Could you check a few things on this model? Use its own coordinates, in mm. A direction names the side the tool comes from. Round coordinates to 2 decimals unless told otherwise and drop trailing zeros. Loops run counter-clockwise (first coordinate to the right, second up) from the corner with the lowest first, then second, coordinate; pieces in that order, holes last.
from build123d import *

# Parameters (mm, degrees)
F1_DEPTH       = 19
F3_D           = 3.4
F3_CSINK_D     = 6.72
F3_CSINK_ANGLE = 90
F5_DEPTH       = 25
F6_R           = 2


with BuildPart() as f1:
    # F0 (on Front) → F1 (new body)
    with BuildSketch(Plane.XZ):
        Polygon((0, 5.0361528993), (0, 0), (40, 0), (40, 10), (35, 10), (35, 5.0361528993), align=None)
    extrude(amount=F1_DEPTH)

    # F3 (through all)
    with Locations(Plane(origin=(0, 0, 0), x_dir=(1, 0, 0), z_dir=(0, 0, -1))):
        with Locations((9, 12), (29, 12)):
            CounterSinkHole(F3_D / 2, F3_CSINK_D / 2, counter_sink_angle=F3_CSINK_ANGLE)

    # F4 (on face) → F5 (cut)
    with BuildSketch(Plane(origin=(0, 0, 0), x_dir=(1, 0, 0), z_dir=(0, 0, -1))):
        Polygon((40, 3.5), (5, 0), (40, 0), align=None)
    extrude(amount=-F5_DEPTH, mode=Mode.SUBTRACT)

    # F6
    f6_edges = [f1.edges().sort_by_distance(p)[0] for p in [
        (40, -11.25, 0),
    ]]
    fillet(f6_edges, radius=F6_R)


solid = f1.part
Item 1: If we section it at D-D, the plane x = 9: Please give me the cut outline in (y, z).
Results list:
outline: (-19, 0) - (-15.36, 0) - (-13.7, 1.66) - (-13.7, 5.04) - (-19, 5.04) - close; (-10.3, 1.66) - (-8.64, 0) - (-0.4, 0) - (-0.4, 5.04) - (-10.3, 5.04) - close
Item 2: Will these pins go through, and if not, where does the flat tip stop? pin 1 (3 mm diameter, centred on y = -9.5, z = 7, fed in from -X); pin 2 (4.5 mm diameter, centred on x = 29, y = -12, fed in from -Z); pin 3 (5.5 mm diameter, centred on x = 19.5, y = -7, fed in from +Z).
Results list:
pin 1: stops at x = 35
pin 2: stops at z = 1.11
pin 3: stops at z = 5.04
Item 3: We'd pull the mould along X, two halves only. Please class faces 3 (the cylindrical face through (27.43, -11.35, 3.37)), 4 (the flat face through (0, -9, 3)), 5 (the flat face through (38, -11, 10)), 6 (the flat face through (40, -11, 6)): released by +X, released by -X, zero draft, split by the parting line, or undercut.
Results list:
face 3: undercut
face 4: released by -X
face 5: zero draft
face 6: released by +X
Item 4: If we section it at B-B, the plane z = 2.5: Please give me the cut outline in (x, y), then the cut area to 3 significant figures.
Results list:
outline: (0, -19) - (40, -19) - (40, -3.5) - (5, 0) - (0, 0) - close; hole circle Ø3.4 at (9, -12); hole circle Ø3.4 at (29, -12)
area: 681 mm2
Item 5: For faces 1 (the flat face through (2, 0, 3)), 2 (the flat face through (18, -9, 5.036)), which set-ups out of +Z, -Z, +X, -X, +Y, -Y let a thin tool reach every point of the face, with its end or its side?
Results list:
face 1: +Z, -Z, +X, -X, +Y
face 2: +Z, -X, +Y, -Y
Item 6: If we section it at A-A, the plane x = 29: Please give me the cut outline in (y, z), then the cut area to 3 significant figures.
Results list:
outline: (-19, 0) - (-15.36, 0) - (-13.7, 1.66) - (-13.7, 5.04) - (-19, 5.04) - close; (-10.3, 1.66) - (-8.64, 0) - (-2.4, 0) - (-2.4, 5.04) - (-10.3, 5.04) - close
area: 63.7 mm2
Item 7: If I drill on line 1 along X through (y, z) = (-12, 3.05); line 2 along Z through (x, y) = (33, -13); line 3 along X through (y, z) = (-10.25, 7.25), over which ranges is the centre line in solid material (lowest first)?
Results list:
line 1: x = 0 to 7.3, 10.7 to 27.3, 30.7 to 40
line 2: z = 0 to 5.04
line 3: x = 35 to 40
Item 8: If we section it at C-C, the plane y = -12: Please give me the cut outline in (x, z), then the cut area to 3 significant figures.
Results list:
outline: (0, 0) - (5.64, 0) - (7.3, 1.66) - (7.3, 5.04) - (0, 5.04) - close; (10.7, 1.66) - (12.36, 0) - (25.64, 0) - (27.3, 1.66) - (27.3, 5.04) - (10.7, 5.04) - close; (30.7, 1.66) - (32.36, 0) - (38, 0) arc R2 ccw to (40, 2) - (40, 10) - (35, 10) - (35, 5.04) - (30.7, 5.04) - close
area: 186 mm2
